Source: CAD feature listing. Evaluate the final solid. Frame: model axes, mm. Face numbers are marked on the shaded views. Coordinates: 2 decimals unless noted, no trailing zeros. Write each loop counter-clockwise with the first axis right and the second up, starting at its lowest first coordinate (ties: lowest second). Pieces come first, ordered by that corner, then holes. Notation, with made-up numbers: M 42.5,-34 L 67.5,-34 A32 cw 67.5,5 Z; hole C 50.25,-33.5 d10. An arc over 180 degrees is marked long. Write item = value, one per line. Start each with the question number.
1. Section query B-B (z = 0). Output: boundary loops of the cut face in (x, y), then the cut area to 3 significant figures.
2. Section query C-C (y = 0.2). Output: boundary loops of the cut face in (x, z), then the cut area to 3 significant figures.
3. Section query A-A (x = 0). Output: boundary loops of the cut face in (y, z).
4. Pull-direction query (X, two-part tool) for the marked faces 1, 2 and 3; classes: pulls with the +X half, pulls with the -X half, needs draft (parallel to the pull), parting line crosses it, or undercut.
5. Line query: line 1 along Z through (x, y) = (0, 0.4); line 2 along X through (y, z) = (-0.85, -2). Output: solid intervals per line, ascending.
6. Pin query (flat end, axial travel): pin 1 Ø1.5 at (y, z) = (-1.5, -0.5) entering from -X; pin 2 Ø4.5 at (x, z) = (0, 0) entering from +Y; pin 3 Ø3 at (y, z) = (1.5, 3.5) entering from +X; pin 4 Ø1 at (x, y) = (4, 1) entering from -Z. Return the tip coordinate at first contact, or that it passes through.
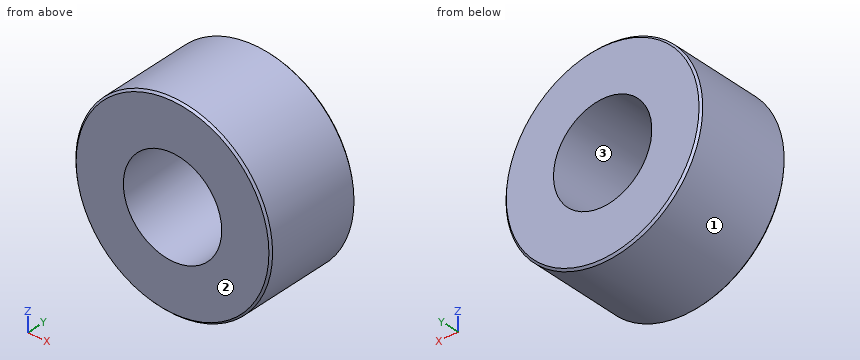
Autodesk Fusion 360 part; units mm, degrees
sketch "Sketch1" plane through (0, 0, 0) normal (0, 1, 0) x (1, 0, 0)
  circle A0 centre (0, 0) radius 5
  circle A1 centre (0, 0) radius 2.5
  dimension "d1" = 10
  dimension "d2" = 5
extrude "Extrude1" add sketch "Sketch1" along normal mid plane 5
chamfer "Chamfer1" distance 0.1 angle 45 2 edges at (-4.6616, -2.5, -1.8081) (-4.6616, 2.5, 1.8081)
Results are:
q1.outline = M -5,-2.4 L -4.9,-2.5 L -2.5,-2.5 L -2.5,2.5 L -4.9,2.5 L -5,2.4 Z; M 2.5,-2.5 L 4.9,-2.5 L 5,-2.4 L 5,2.4 L 4.9,2.5 L 2.5,2.5 Z
q1.area = 25.0 mm^2
q2.outline = C 0,0 d10; hole C 0,0 d5
q2.area = 58.9 mm^2
q3.outline = M -2.5,-4.9 L -2.4,-5 L 2.4,-5 L 2.5,-4.9 L 2.5,-2.5 L -2.5,-2.5 Z; M -2.5,2.5 L 2.5,2.5 L 2.5,4.9 L 2.4,5 L -2.4,5 L -2.5,4.9 Z
q4.face_1 = parting line crosses it
q4.face_2 = needs draft
q4.face_3 = undercut
q5.line_1 = -5 to -2.5, 2.5 to 5
q5.line_2 = -4.58 to -1.5, 1.5 to 4.58
q6.pin_1 = -5
q6.pin_2 = through
q6.pin_3 = 4.58
q6.pin_4 = -3.57
